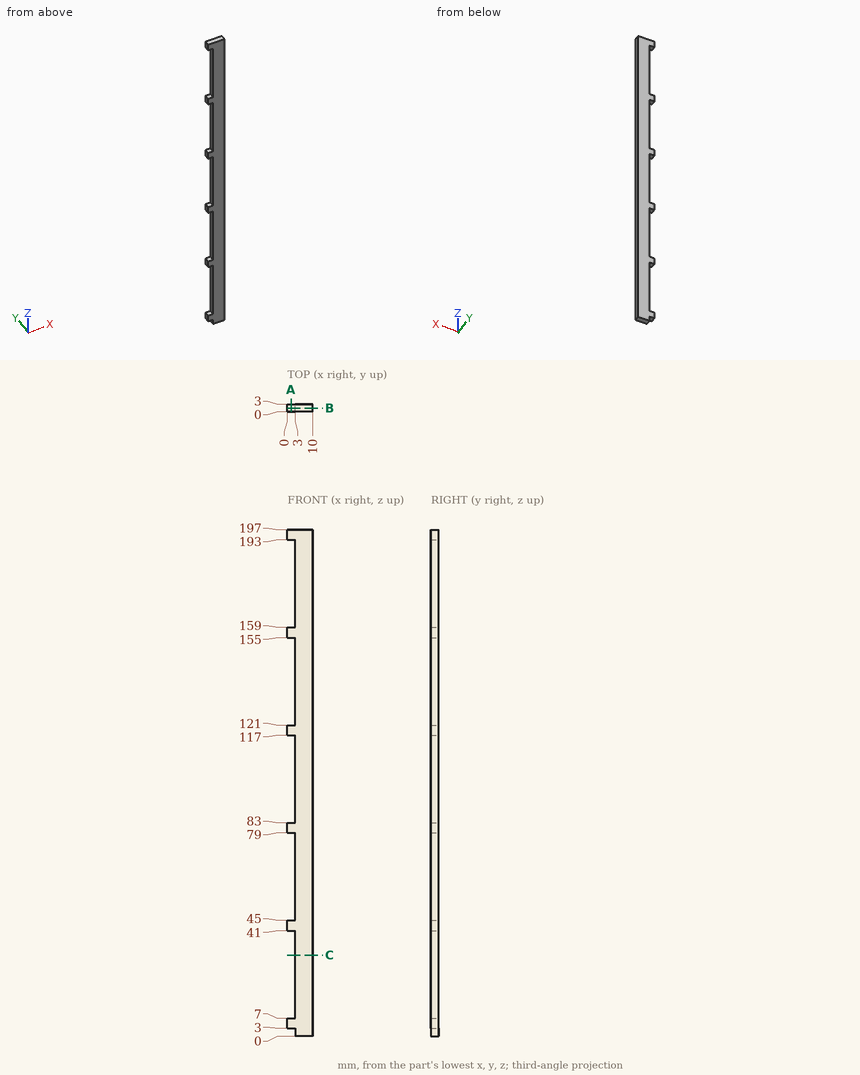
Drawing for the job (mm, zero at the part's lowest x, y, z). Round coordinates to 2 decimals unless told otherwise and drop trailing zeros. Loops run counter-clockwise (first coordinate to the right, second up) from the corner with the lowest first, then second, coordinate; pieces in that order, holes last. Notation, with made-up numbers: (-36.75, 9.5) -> (9.25, 9.5) arc R10 ccw to (9.25, 27.5) -> close; hole circle Ø2 at (-21, 69). An arc over 180 degrees is marked (long way). Answer in a Markdown table with one row per item.
Item 1: Saw through at B-B (y = 1.4). Write the cut outline in (x, z), and give its area (3 significant figures).
Answers below:
| item | result |
|---|---|
| outline | (0, 3) -> (3, 3) -> (3, 0) -> (10, 0) -> (10, 197) -> (0, 197) -> (0, 193) -> (3, 193) -> (3, 159) -> (0, 159) -> (0, 155) -> (3, 155) -> (3, 121) -> (0, 121) -> (0, 117) -> (3, 117) -> (3, 83) -> (0, 83) -> (0, 79) -> (3, 79) -> (3, 45) -> (0, 45) -> (0, 41) -> (3, 41) -> (3, 7) -> (0, 7) -> close |
| area | 1,450 mm² |
Item 2: Saw through at C-C (z = 31.5). Write the cut outline in (x, y).
Answers below:
| item | result |
|---|---|
| outline | (3, 0) -> (10, 0) -> (10, 3) -> (3, 3) -> close |
Item 3: Drill centre lines: L1, parallel to Z at x = 1.75, y = 1.9; L2, parallel to X at y = 2.25, z = 75.5. Where is each one in solid material? Low to high. Write a range as [from, to].
Answers below:
| item | result |
|---|---|
| L1 | z = [3, 7], [41, 45], [79, 83], [117, 121], [155, 159], [193, 197] |
| L2 | x = [3, 10] |
Item 4: Saw through at A-A (x = 1.5). Write the cut outline in (y, z).
Answers below:
| item | result |
|---|---|
| outline | (0, 3) -> (3, 3) -> (3, 7) -> (0, 7) -> close; (0, 41) -> (3, 41) -> (3, 45) -> (0, 45) -> close; (0, 79) -> (3, 79) -> (3, 83) -> (0, 83) -> close; (0, 117) -> (3, 117) -> (3, 121) -> (0, 121) -> close; (0, 155) -> (3, 155) -> (3, 159) -> (0, 159) -> close; (0, 193) -> (3, 193) -> (3, 197) -> (0, 197) -> close |
Item 5: Pin check, flat tips, straight feed: pin 1 (0.9 mm diameter, centred on y = 1, z = 1.5, fed in from -X); pin 2 (1.5 mm diameter, centred on x = 2, y = 1, fed in from -Z); pin 3 (1.5 mm diameter, centred on x = 2.5, z = 24, fed in from +Y). Stop position of each tip, or through.
Answers below:
| item | result |
|---|---|
| pin 1 | stops at x = 3 |
| pin 2 | stops at z = 3 |
| pin 3 | stops at y = 3 |
